The listing builds one solid part. Answer for the finished solid, in the listing's coordinates (mm). A direction names the side the tool comes from. Give positions to 0.01 mm unless a question says otherwise; leave off trailing zeros. Order: outer loops, then holes, each group sorted by start corner. A loop starts at its lowest first (then second) coordinate and runs counter-clockwise, first axis right, second up. Notation, with made-up numbers: (-15, -15) - (33, -15) arc R21 cw to (33, 5) - close; hole circle Ø2 at (-4.5, 7.25). An arc over 180 degrees is marked (long way). Answer in a Markdown table with one row per item.
from build123d import *

# Parameters (mm, degrees)
SKETCH_1_W          = 320
SKETCH_1_H          = 300
EXTRUDE_1_DEPTH     = 10
CHAMFER_1_SIZE      = 10
CUT_EXTRUDE_1_REACH = 221.545
CHAMFER_2_SIZE      = 8


with BuildPart() as part:
    # 草图1 → 凸台-拉伸1 (new body)
    with BuildSketch(Plane.XY):
        Rectangle(SKETCH_1_W, SKETCH_1_H)
    extrude(amount=EXTRUDE_1_DEPTH)

    # 倒角1
    chamfer_1_edges = [part.edges().sort_by_distance(p)[0] for p in [
        (160, -150, 5),
        (-160, -150, 5),
        (-160, 150, 5),
        (160, 150, 5),
    ]]
    chamfer(chamfer_1_edges, length=CHAMFER_1_SIZE)

    # 草图2 → 切除-拉伸1 (cut, up to next)
    with BuildSketch(Plane.XY.offset(10), mode=Mode.PRIVATE) as cut_extrude_1_sk1:
        with BuildLine():
            Line((-130, 125), (130, 125))
            ThreePointArc((130, 125), (133.535533906, 123.535533906), (135, 120))
            Line((135, 120), (135, -120))
            ThreePointArc((135, -120), (133.535533906, -123.535533906), (130, -125))
            Line((130, -125), (-130, -125))
            ThreePointArc((-130, -125), (-133.535533906, -123.535533906), (-135, -120))
            Line((-135, -120), (-135, 120))
            ThreePointArc((-135, 120), (-133.535533906, 123.535533906), (-130, 125))
        make_face()
    cut_extrude_1_tool1 = extrude(cut_extrude_1_sk1.sketch, amount=-CUT_EXTRUDE_1_REACH, mode=Mode.PRIVATE) & part.part
    add(cut_extrude_1_tool1.solids().sort_by_distance((0, 0, 10))[0], mode=Mode.SUBTRACT)

    # 倒角2
    chamfer_2_edges = [part.edges().sort_by_distance(p)[0] for p in [
        (-133.535533906, -123.535533906, 10),
        (0, -125, 10),
        (133.535533906, -123.535533906, 10),
        (135, 0, 10),
        (133.535533906, 123.535533906, 10),
        (0, 125, 10),
        (-133.535533906, 123.535533906, 10),
        (-135, 0, 10),
    ]]
    chamfer(chamfer_2_edges, length=CHAMFER_2_SIZE)


solid = part.part
Item 1: Consider line 1 (Y direction, x = -22, z = 0.5); line 2 (X direction, y = 64.5, z = 1.5); line 3 (Y direction, x = -45, z = 7.25). Determine where each line is inside the solid, lowest interval first.
Answer block:
| item | result |
|---|---|
| line 1 | -150 to -125, 125 to 150 |
| line 2 | -160 to -135, 135 to 160 |
| line 3 | -150 to -130.25, 130.25 to 150 |
Item 2: Determine the mould class of faces 1 (the face through (-160, -2, 5)), 2 (the face through (139, 2, 6)), 3 (the face through (-139, -2, 6)), 4 (the face through (160, -2, 5)) for opening direction X: pulls with the +X half, pulls with the -X half, needs draft (parallel to the pull), parting line crosses it, or undercut.
Answer block:
| item | result |
|---|---|
| face 1 | pulls with the -X half |
| face 2 | undercut |
| face 3 | undercut |
| face 4 | pulls with the +X half |
Item 3: Find section A-A on x = 96. Write down the section's boundary in (y, z).
Answer block:
| item | result |
|---|---|
| outline | (-150, 0) - (-125, 0) - (-125, 2) - (-133, 10) - (-150, 10) - close; (125, 0) - (150, 0) - (150, 10) - (133, 10) - (125, 2) - close |
Item 4: Find section B-B on y = -115.5. Write down the section's boundary in (x, z).
Answer block:
| item | result |
|---|---|
| outline | (-160, 0) - (-135, 0) - (-135, 2) - (-143, 10) - (-160, 10) - close; (135, 0) - (160, 0) - (160, 10) - (143, 10) - (135, 2) - close |
Item 5: Find section C-C on z = 4.25. Write down the section's boundary in (x, y).
Answer block:
| item | result |
|---|---|
| outline | (-160, -140) - (-150, -150) - (150, -150) - (160, -140) - (160, 140) - (150, 150) - (-150, 150) - (-160, 140) - close; hole (-137.25, -120) arc R7.25 ccw to (-130, -127.25) - (130, -127.25) arc R7.25 ccw to (137.25, -120) - (137.25, 120) arc R7.25 ccw to (130, 127.25) - (-130, 127.25) arc R7.25 ccw to (-137.25, 120) - close |
Item 6: Which of the six approach directions +Z, -Z, +X, -X, +Y, -Y give full straight-line access (tool end or side, diameter ignored) to faces 5 (the face through (-155, -145, 5)), 6 (the face through (136.39, -126.25, 5.94))?
Answer block:
| item | result |
|---|---|
| face 5 | +Z, -Z, -X, -Y |
| face 6 | +Z |
